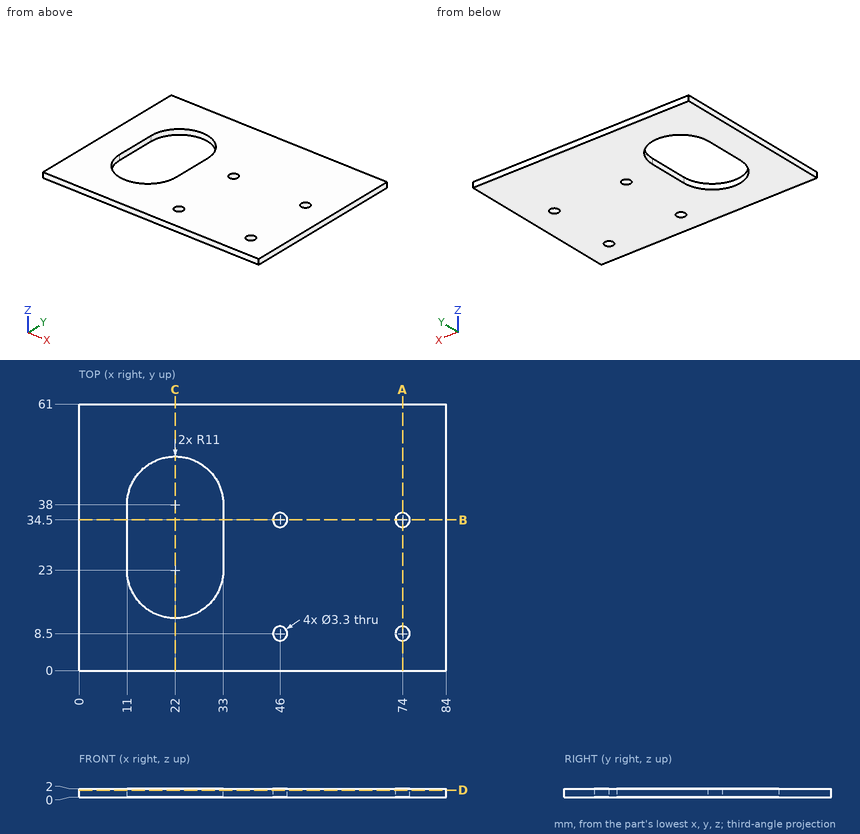
Answer from the drawing. Dimensions are ordinates in mm from the lowest x, y and z of the part. Coordinates: 2 decimals unless noted, no trailing zeros. Write each loop counter-clockwise with the first axis right and the second up, starting at its lowest first coordinate (ties: lowest second). Pieces come first, ordered by that corner, then holes. Notation, with made-up numbers: M 65,5 L 89,5 A27 cw 89,23 Z; hole C -8,7.25 d4. An arc over 180 degrees is marked long. Use one line per item in the form item = value. Start each with the question number.
1. Straight lines are drawn through the part: probe 1 along Y at (x, z) = (46, 1.3); probe 2 along X at (y, z) = (8.5, 0.9); probe 3 along X at (y, z) = (24.5, 0.9). For each, find the intervals that lie inside material, in ascending order. Write a range as from..to.
2. The part is cut by section C-C (x = 22). Give the vertices of the cut face in (y, z).
3. The part is cut by section B-B (y = 34.5). Give the vertices of the cut face in (x, z).
4. This flat-tipped pin is pushed along its axis until it touches: P1, Ø2.5, axis at x = 74, y = 34.5, coming from the +Z side. Where does it stop, or does it pass through?
5. The part is cut by section D-D (z = 1.65). Give the vertices of the cut face in (x, y).
6. The part is cut by section A-A (x = 74). Give the vertices of the cut face in (y, z), plus the area to 3 significant figures.
Evaluation:
q1.probe_1 = 0..6.85, 10.15..32.85, 36.15..61
q1.probe_2 = 0..44.35, 47.65..72.35, 75.65..84
q1.probe_3 = 0..11, 33..84
q2.outline = M 0,0 L 12,0 L 12,2 L 0,2 Z; M 49,0 L 61,0 L 61,2 L 49,2 Z
q3.outline = M 0,0 L 11,0 L 11,2 L 0,2 Z; M 33,0 L 44.35,0 L 44.35,2 L 33,2 Z; M 47.65,0 L 72.35,0 L 72.35,2 L 47.65,2 Z; M 75.65,0 L 84,0 L 84,2 L 75.65,2 Z
q4.P1 = through
q5.outline = M 0,0 L 84,0 L 84,61 L 0,61 Z; hole M 11,23 A11 ccw 33,23 L 33,38 A11 ccw 11,38 Z; hole C 46,8.5 d3.3; hole C 46,34.5 d3.3; hole C 74,8.5 d3.3; hole C 74,34.5 d3.3
q6.outline = M 0,0 L 6.85,0 L 6.85,2 L 0,2 Z; M 10.15,0 L 32.85,0 L 32.85,2 L 10.15,2 Z; M 36.15,0 L 61,0 L 61,2 L 36.15,2 Z
q6.area = 109 mm^2
